Build history of the part. All positions in model axes, mm. Face numbers are marked on the shaded views. A direction names the side the tool comes from. Give positions to 0.01 mm unless a question says otherwise; leave off trailing zeros. Loops run counter-clockwise (first coordinate to the right, second up) from the corner with the lowest first, then second, coordinate; pieces in that order, holes last. Notation, with made-up numbers: (32, -0.5) -> (62, -0.5) arc R32 cw to (62, 38.5) -> close; hole circle Ø2 at (41, 2). An arc over 180 degrees is marked (long way). Answer in a Markdown table with one row per item. Add a question column.
from build123d import *

# Parameters (mm, degrees)
SKETCH1_W           = 400
SKETCH1_H           = 400
BOSS_EXTRUDE1_DEPTH = 200
SKETCH2_W           = 370
SKETCH2_H           = 370
CUT_EXTRUDE1_DEPTH  = 150
FILLET1_R           = 10
CHAMFER1_SIZE       = 10
CUT_EXTRUDE2_REACH  = 491.898
CUT_EXTRUDE3_DEPTH  = 40


with BuildPart() as part:
    # Sketch1 → Boss-Extrude1 (new body)
    with BuildSketch(Plane(origin=(0, 0, 0), x_dir=(1, 0, 0), z_dir=(0, 1, 0))):
        Rectangle(SKETCH1_W, SKETCH1_H)
    extrude(amount=BOSS_EXTRUDE1_DEPTH)

    # Sketch2 → Cut-Extrude1 (cut)
    with BuildSketch(Plane(origin=(0, 200, 0), x_dir=(1, 0, 0), z_dir=(0, 1, 0))):
        Rectangle(SKETCH2_W, SKETCH2_H)
    extrude(amount=-CUT_EXTRUDE1_DEPTH, mode=Mode.SUBTRACT)

    # Fillet1
    fillet1_edges = [part.edges().sort_by_distance(p)[0] for p in [
        (-185, 50, 0),
        (-185, 125, 185),
        (0, 50, -185),
        (-185, 125, -185),
        (185, 50, 0),
        (185, 125, -185),
        (0, 50, 185),
        (185, 125, 185),
    ]]
    fillet(fillet1_edges, radius=FILLET1_R)

    # Chamfer1
    chamfer1_edges = [part.edges().sort_by_distance(p)[0] for p in [
        (0, 200, -185),
        (185, 200, 0),
        (0, 200, 185),
        (-185, 200, 0),
        (182.071067812, 200, 182.071067812),
        (-182.071067812, 200, 182.071067812),
        (182.071067812, 200, -182.071067812),
        (-182.071067812, 200, -182.071067812),
        (-200, 100, -200),
        (200, 100, -200),
        (200, 100, 200),
        (-200, 100, 200),
    ]]
    chamfer(chamfer1_edges, length=CHAMFER1_SIZE)

    # Sketch3 → Cut-Extrude2 (cut, up to next)
    with BuildSketch(Plane.XY.offset(200), mode=Mode.PRIVATE) as cut_extrude2_sk1:
        with BuildLine():
            Line((-72, 60), (72, 60))
            ThreePointArc((72, 60), (74.121320344, 59.121320344), (75, 57))
            Line((75, 57), (75, 53))
            ThreePointArc((75, 53), (74.121320344, 50.878679656), (72, 50))
            Line((72, 50), (-72, 50))
            ThreePointArc((-72, 50), (-74.121320344, 50.878679656), (-75, 53))
            Line((-75, 53), (-75, 57))
            ThreePointArc((-75, 57), (-74.121320344, 59.121320344), (-72, 60))
        make_face()
    cut_extrude2_tool1 = extrude(cut_extrude2_sk1.sketch, amount=-CUT_EXTRUDE2_REACH, mode=Mode.PRIVATE) & part.part
    add(cut_extrude2_tool1.solids().sort_by_distance((0, 55, 200))[0], mode=Mode.SUBTRACT)

    # Sketch4 → Cut-Extrude3 (cut)
    with BuildSketch(Plane.XZ):
        Polygon((190, 125), (135, 125), (125, 135), (125, 190), (135, 200), (-135, 200), (-125, 190), (-125, 135), (-135, 125), (-190, 125), (-200, 135), (-200, -135), (-190, -125), (-135, -125), (-125, -135), (-125, -190), (-135, -200), (135, -200), (125, -190), (125, -135), (135, -125), (190, -125), (200, -135), (200, 135), align=None)
    extrude(amount=-CUT_EXTRUDE3_DEPTH, mode=Mode.SUBTRACT)


solid = part.part
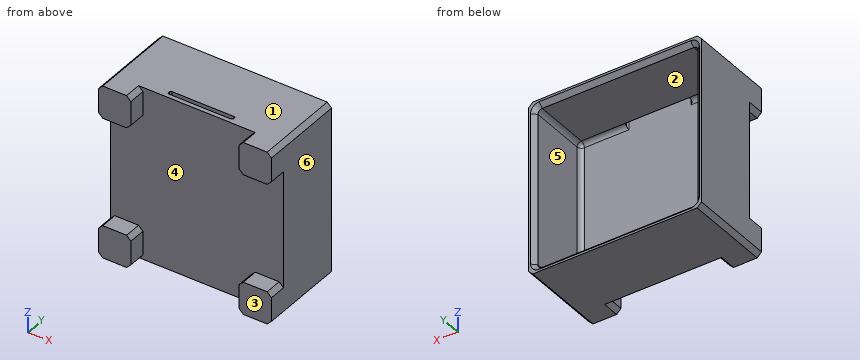
(1) Saw through at C-C, the plane z = 158.5. List the corners of the cut face in (x, y), then the cut area to 3 significant figures.
(2) Flat gauge pins, fed straight in: pin 1 Ø10 at (x, z) = (-43, 138.5) entering from +Y; pin 2 Ø12 at (x, z) = (-115, 128) entering from -Y. Where does each tip first touch, or does it go through?
(3) 3-axis set-ups, long thin cutter, end or side, ignore diameter. For the marked faces 4, 5 and 6: which of +Z, -Z, +X, -X, +Y, -Y reach the whole face in a straight line?
(4) Saw through at B-B, the plane x = -33.5. List the corners of the cut face in (y, z).
(5) Saw through at A-A, the plane y = 24. State how many separate pieces and enclosed holes the cut face has, then the cut area to 3 significant figures.
(6) Wall check: line 1 along X through (y, z) = (78, -54); line 2 along X through (y, z) = (33.5, -161.5). Give the ranges that are in metal, low to high. Write a range as from..to.
(7) Two-plate mould, pull along Z, no slides. Class the marked faces 1, 2 and 3: released by +Z, released by -Z, zero draft, split by the parting line, or undercut.
(8) Saw through at D-D, the plane y = 172. List the corners of the cut face in (x, z).
Worked answers:
| question | item | result |
|---|---|---|
| 1 | outline | (-200, 0) -> (-125, 0) -> (-125, 40) -> (125, 40) -> (125, 0) -> (200, 0) -> (200, 200) -> (195, 200) -> (185, 190) -> (185, 60) arc R10 cw to (175, 50) -> (-175, 50) arc R10 cw to (-185, 60) -> (-185, 190) -> (-195, 200) -> (-200, 200) -> close |
| 1 | area | 14,400 mm^2 |
| 2 | pin 1 | y = 50 |
| 2 | pin 2 | y = 40 |
| 3 | face 4 | -Y |
| 3 | face 5 | +Y |
| 3 | face 6 | +Z, -Z, +X, +Y, -Y |
| 4 | outline | (40, -200) -> (200, -200) -> (200, -195) -> (190, -185) -> (60, -185) arc R10 cw to (50, -175) -> (50, 200) -> (40, 200) -> close; (60, 185) -> (190, 185) -> (200, 195) -> (200, 200) -> (60, 200) -> close |
| 5 | separate pieces | 4 |
| 5 | enclosed holes | 0 |
| 5 | area | 21,700 mm^2 |
| 6 | line 1 | -200..-185, 185..200 |
| 6 | line 2 | -200..-125, 125..200 |
| 7 | face 1 | released by +Z |
| 7 | face 2 | undercut |
| 7 | face 3 | zero draft |
| 8 | outline | (-200, -190) -> (-190, -200) -> (190, -200) -> (200, -190) -> (200, 190) -> (190, 200) -> (-190, 200) -> (-200, 190) -> close; hole (-185, -175) arc R10 ccw to (-175, -185) -> (175, -185) arc R10 ccw to (185, -175) -> (185, 175) arc R10 ccw to (175, 185) -> (-175, 185) arc R10 ccw to (-185, 175) -> close |
